from build123d import *

# Parameters (mm, degrees)
BOSS_EXTRUDE1_DEPTH      = 13.5
BOSS_EXTRUDE2_DEPTH      = 18.5
BOSS_EXTRUDE3_DEPTH      = 5
SKETCH4_W                = 45.922011884
SKETCH4_H                = 20
BOSS_EXTRUDE4_DEPTH      = 13.5
SKETCH2_R                = 4
CUT_EXTRUDE1_DEPTH       = 268.629329099
SKETCH5_R                = 8
CUT_EXTRUDE2_DEPTH       = 4
SKETCH6_R                = 9
CUT_EXTRUDE3_DEPTH       = 12
SKETCH7_R                = 12.5
CUT_EXTRUDE4_DEPTH       = 5
BOSS_EXTRUDE5_DEPTH      = 13.5
CUT_EXTRUDE5_REACH       = 210.1
CUT_EXTRUDE5_END_RADIUS  = 45
SKETCH8_R                = 9
CUT_EXTRUDE6_REACH       = 210.1
SKETCH10_R               = 4.5
SKETCH18_R               = 11
CUT_EXTRUDE9_DEPTH       = 47
CUT_EXTRUDE10_DEPTH      = 268.629329099
CUT_EXTRUDE10_DEPTH_BACK = 268.629329099
SKETCH19_W               = 45.922011884
SKETCH19_H               = 198
M6_CLEARANCE_HOLE1_D     = 6.6
SKETCH30_R               = 8.025
CUT_EXTRUDE13_DEPTH      = 4
BOSS_EXTRUDE9_DEPTH      = 16
M5_TAPPED_HOLE2_D        = 4.2
CUT_EXTRUDE16_DEPTH      = 3
M2_TAPPED_HOLE1_D        = 1.6
M2_TAPPED_HOLE1_DEPTH    = 8
M2_TAPPED_HOLE1_TIP      = 0.480688495


with BuildPart() as part:
    # Sketch1 → Boss-Extrude1 (new, symmetric)
    with BuildSketch(Plane(origin=(0, 0, 0), x_dir=(1, 0, 0), z_dir=(0, 1, 0))):
        with BuildLine():
            ThreePointArc((17.220754456, -41.574578963), (0, -45), (-17.220754456, -41.574578963))
            Line((-17.220754456, -41.574578963), (-22.961005942, -55.432771951))
            ThreePointArc((-22.961005942, -55.432771951), (0, -60), (22.961005942, -55.432771951))
            Line((22.961005942, -55.432771951), (17.220754456, -41.574578963))
        make_face()
    extrude(amount=BOSS_EXTRUDE1_DEPTH, both=True)

    # Sketch1_3 → Boss-Extrude2 (add, symmetric)
    with BuildSketch(Plane(origin=(0, 0, 0), x_dir=(1, 0, 0), z_dir=(0, 1, 0))):
        with BuildLine():
            ThreePointArc((19.134171618, -46.193976626), (0, -50), (-19.134171618, -46.193976626))
            Line((-19.134171618, -46.193976626), (-21.04758878, -50.813374288))
            ThreePointArc((-21.04758878, -50.813374288), (0, -55), (21.04758878, -50.813374288))
            Line((21.04758878, -50.813374288), (19.134171618, -46.193976626))
        make_face()
    extrude(amount=BOSS_EXTRUDE2_DEPTH, both=True)

    # Sketch3 → Boss-Extrude3 (add, symmetric)
    with BuildSketch(Plane.XZ):
        with BuildLine():
            Line((-22.961005942, 266), (-22.961005942, 55.432771951))
            ThreePointArc((-22.961005942, 55.432771951), (-20.481139434, 56.39612511), (-17.961005942, 57.248600555))
            Line((-17.961005942, 57.248600555), (-17.961005942, 246))
            Line((-17.961005942, 246), (17.961005942, 246))
            Line((17.961005942, 246), (17.961005942, 57.248600555))
            ThreePointArc((17.961005942, 57.248600555), (20.481139434, 56.39612511), (22.961005942, 55.432771951))
            Line((22.961005942, 55.432771951), (22.961005942, 266))
            Line((22.961005942, 266), (-22.961005942, 266))
        make_face()
    extrude(amount=BOSS_EXTRUDE3_DEPTH, both=True)

    # Sketch4 → Boss-Extrude4 (add, symmetric)
    with BuildSketch(Plane(origin=(0, 0, 0), x_dir=(1, 0, 0), z_dir=(0, 1, 0))):
        with Locations((0, -256)):
            Rectangle(SKETCH4_W, SKETCH4_H)
    extrude(amount=BOSS_EXTRUDE4_DEPTH, both=True)

    # Sketch2 → Cut-Extrude1 (cut, through all)
    with BuildSketch(Plane.XY):
        with Locations(Location((0, 0, 0), (0, 0, 180))):
            Circle(SKETCH2_R)
    extrude(amount=CUT_EXTRUDE1_DEPTH, mode=Mode.SUBTRACT)

    # Sketch5 → Cut-Extrude2 (cut)
    with BuildSketch(Plane(origin=(0, 0, 246), x_dir=(-1, 0, 0), z_dir=(0, 0, -1))):
        Circle(SKETCH5_R)
    extrude(amount=-CUT_EXTRUDE2_DEPTH, mode=Mode.SUBTRACT)

    # Sketch6 → Cut-Extrude3 (cut)
    with BuildSketch(Plane.XY.offset(266)):
        Circle(SKETCH6_R)
    extrude(amount=-CUT_EXTRUDE3_DEPTH, mode=Mode.SUBTRACT)

    # Sketch7 → Cut-Extrude4 (cut)
    with BuildSketch(Plane.XY.offset(266)):
        Circle(SKETCH7_R)
    extrude(amount=-CUT_EXTRUDE4_DEPTH, mode=Mode.SUBTRACT)

    # Sketch9 → Boss-Extrude5 (add, symmetric)
    with BuildSketch(Plane(origin=(0, 0, 0), x_dir=(1, 0, 0), z_dir=(0, 1, 0))):
        with BuildLine():
            Line((-22.961005942, -55.432771951), (-22.961005942, -68))
            Line((-22.961005942, -68), (22.961005942, -68))
            Line((22.961005942, -68), (22.961005942, -55.432771951))
            ThreePointArc((22.961005942, -55.432771951), (0, -60), (-22.961005942, -55.432771951))
        make_face()
    extrude(amount=BOSS_EXTRUDE5_DEPTH, both=True)

    # Cut-Extrude5: up to this cylinder (the profile starts outside it)
    cut_extrude5_end = Plane(origin=(0, 0, 0), z_dir=(0, -1, 0)) * Cylinder(CUT_EXTRUDE5_END_RADIUS, 511.2, mode=Mode.PRIVATE)
    # Sketch8 → Cut-Extrude5 (cut, up to the surface)
    with BuildSketch(Plane.XY.offset(60), mode=Mode.PRIVATE) as cut_extrude5_sk1:
        Circle(SKETCH8_R)
    cut_extrude5_tool1 = extrude(cut_extrude5_sk1.sketch, amount=-CUT_EXTRUDE5_REACH, mode=Mode.PRIVATE) - cut_extrude5_end
    add(cut_extrude5_tool1.solids().sort_by_distance((0, 0, 60))[0], mode=Mode.SUBTRACT)

    # Sketch10 → Cut-Extrude6 (cut, up to next)
    with BuildSketch(Plane.XY.offset(60), mode=Mode.PRIVATE) as cut_extrude6_sk1:
        with Locations(Location((0, 0, 0), (0, 0, 180))):
            Circle(SKETCH10_R)
    cut_extrude6_tool1 = extrude(cut_extrude6_sk1.sketch, amount=CUT_EXTRUDE6_REACH, mode=Mode.PRIVATE) & part.part
    add(cut_extrude6_tool1.solids().sort_by_distance((0, 0, 60))[0], mode=Mode.SUBTRACT)

    # Sketch18 → Cut-Extrude9 (cut)
    with BuildSketch(Plane.XY):
        with Locations(Location((0, 0, 0), (0, 0, 180))):
            Circle(SKETCH18_R)
    extrude(amount=CUT_EXTRUDE9_DEPTH, mode=Mode.SUBTRACT)

    # Sketch19 → Cut-Extrude10 (cut, two sides: drawn at the far end of the back side and taken through both)
    with BuildSketch(Plane(origin=(0, 0, 0), x_dir=(1, 0, 0), z_dir=(0, 1, 0)).offset(-CUT_EXTRUDE10_DEPTH_BACK)):
        with Locations((0, -167)):
            Rectangle(SKETCH19_W, SKETCH19_H)
    extrude(amount=CUT_EXTRUDE10_DEPTH + CUT_EXTRUDE10_DEPTH_BACK, mode=Mode.SUBTRACT)

    # Sketch23 → M5 Tapped Hole1 (revolve, cut)
    with BuildSketch(Plane(origin=(14.26606865, 8, 68), x_dir=(0, -1, 0), z_dir=(1, 0, 0))):
        Polygon((0, 0), (0, 11.3618073), (2.1, 10.1), (2.1, 0), align=None)
    m5_tapped_hole1 = revolve(axis=Axis((14.26606865, 8, 74.35), (0, 0, -1)), mode=Mode.SUBTRACT)

    # Mirror1: M5 Tapped Hole1 across plane
    add(m5_tapped_hole1.mirror(Plane(origin=(0, 0, 0), x_dir=(0, 0, 1), z_dir=(1, 0, 0))), mode=Mode.SUBTRACT)

    # M6 Clearance Hole1 (through all)
    with Locations(Plane(origin=(0, 18.5, 0), x_dir=(1, 0, 0), z_dir=(0, 1, 0))):
        with Locations((-13.587999868, -50.71110588), (13.587999868, -50.71110588)):
            Hole(M6_CLEARANCE_HOLE1_D / 2)

    # Sketch30 → Cut-Extrude13 (cut)
    with BuildSketch(Plane(origin=(0, 0, 60), x_dir=(-1, 0, 0), z_dir=(0, 0, -1))):
        Circle(SKETCH30_R)
    extrude(amount=-CUT_EXTRUDE13_DEPTH, mode=Mode.SUBTRACT)

    # Sketch37 → Boss-Extrude9 (add)
    with BuildSketch(Plane.XZ.offset(13.5)):
        with BuildLine():
            Line((-22.961005942, 68), (22.961005942, 68))
            Line((22.961005942, 68), (22.961005942, 57))
            ThreePointArc((22.961005942, 57), (0, 61.450856738), (-22.961005942, 57))
            Line((-22.961005942, 57), (-22.961005942, 68))
        make_face()
    extrude(amount=BOSS_EXTRUDE9_DEPTH)

    # M5 Tapped Hole2 (through all)
    with Locations(Plane.XY.offset(68)):
        with Locations((-14.26606865, -24), (14.26606865, -24)):
            Hole(M5_TAPPED_HOLE2_D / 2)

    # Sketch41 → Cut-Extrude16 (cut)
    with BuildSketch(Plane.XY.offset(68)):
        with BuildLine():
            Line((-7, 13.5), (-7, 8))
            ThreePointArc((-7, 8), (-6.560660172, 6.939339828), (-5.5, 6.5))
            Line((-5.5, 6.5), (5.5, 6.5))
            ThreePointArc((5.5, 6.5), (6.560660172, 6.939339828), (7, 8))
            Line((7, 8), (7, 13.5))
            Line((7, 13.5), (-7, 13.5))
        make_face()
    extrude(amount=-CUT_EXTRUDE16_DEPTH, mode=Mode.SUBTRACT)

    # M2 Tapped Hole1
    with Locations(Plane.XY.offset(65)):
        with Locations((-5, 10.5), (5, 10.5)):
            Hole(M2_TAPPED_HOLE1_D / 2, depth=M2_TAPPED_HOLE1_DEPTH)
            with Locations((0, 0, -(M2_TAPPED_HOLE1_DEPTH + M2_TAPPED_HOLE1_TIP / 2))):  # 118° drill point
                Cone(0, M2_TAPPED_HOLE1_D / 2, M2_TAPPED_HOLE1_TIP, mode=Mode.SUBTRACT)


solid = part.part
Geometry check sheet. Reference: the model listing, model coordinates, mm. A direction names the side the tool comes from. Coordinates: 2 decimals unless noted, no trailing zeros. Loops run counter-clockwise (first coordinate to the right, second up) from the corner with the lowest first, then second, coordinate; pieces in that order, holes last. Notation, with made-up numbers: (-25, 69.25) - (22, 69.25) arc R12 cw to (22, 84.25) - close; hole circle Ø1 at (73, -11.5). An arc over 180 degrees is marked (long way). Use one line per item in the form item = value. Start each with the question number.
Item 1: Section check C-C, the plane y = -6. Enter the section's corners in (x, z), and give its area (3 significant figures).
Item 2: Section check B-B, the plane y = -1. Enter the section's corners in (x, z), and give its area (3 significant figures).
Item 3: Section check D-D, the plane y = -24. Enter the section's corners in (x, z).
Item 4: Gauge pin test, flat ends, axial feed: pin 1 (10.5 mm diameter, centred on x = 0, y = 0, fed in from -Z); pin 2 (1.8 mm diameter, centred on x = -17, z = 50.5, fed in from -Y); pin 3 (4 mm diameter, centred on y = 9, z = 44.5, fed in from +X); pin 4 (5 mm diameter, centred on x = -14.27, y = -24, fed in from +Z). Record the tip position at first contact, or that the pin passes through.
Item 5: Mould release check, pull along Y, two halves, no side actions. Record for faces 1 (the face through (0, -18.5, 53)), 2 (the face through (16.364, -23.908, 63.549)), 3 (the face through (0, -16, 50)): +Y half, -Y half, draft (parallel to the pull), parting line (faces both ways), or undercut.
Item 6: Thickness scan on probe 1 along X at (y, z) = (10.5, 61); probe 2 along X at (y, z) = (-6, 48.5); probe 3 along Y at (x, z) = (5, 59.5). Record the ranges inside material, lowest first.
Item 7: Tool access check on faces 4 (the face through (6.55, 6.93, 66.52)), 5 (the face through (-2, 9, 47)), 6 (the face through (14.2, 10.1, 63)), 7 (the face through (18.687, -15.965, 51.728)). Record the directions out of +Z, -Z, +X, -X, +Y, -Y that give a thin tool (end or side, any length) a straight path to the whole face; none if there is none.
Computed:
q1.outline = (-22.96, 55.43) - (-17.22, 41.57) arc R45 cw to (-9.22, 44.05) - (-9.22, 47) - (-6.71, 47) - (-6.71, 60) - (-5.33, 60) - (-5.33, 64) - (5.33, 64) - (5.33, 60) - (6.71, 60) - (6.71, 47) - (9.22, 47) - (9.22, 44.05) arc R45 cw to (17.22, 41.57) - (22.96, 55.43) - (22.96, 68) - (-22.96, 68) - close; hole circle Ø6.6 at (-13.59, 50.71); hole circle Ø6.6 at (13.59, 50.71)
q1.area = 726 mm2
q2.outline = (-22.96, 55.43) - (-17.22, 41.57) arc R45 cw to (-10.95, 43.65) - (-10.95, 47) - (-8.94, 47) - (-8.94, 60) - (-7.96, 60) - (-7.96, 64) - (-4.39, 64) - (-4.39, 68) - (-22.96, 68) - close; (4.39, 64) - (7.96, 64) - (7.96, 60) - (8.94, 60) - (8.94, 47) - (10.95, 47) - (10.95, 43.65) arc R45 cw to (17.22, 41.57) - (22.96, 55.43) - (22.96, 68) - (4.39, 68) - close; hole circle Ø6.6 at (-13.59, 50.71); hole circle Ø6.6 at (13.59, 50.71)
q2.area = 601 mm2
q3.outline = (-22.96, 57) arc R61.45 cw to (-16.37, 59.23) - (-16.37, 68) - (-22.96, 68) - close; (-12.17, 60.23) arc R61.45 cw to (12.17, 60.23) - (12.17, 68) - (-12.17, 68) - close; (16.37, 59.23) arc R61.45 cw to (22.96, 57) - (22.96, 68) - (16.37, 68) - close
q4.pin_1 = 64
q4.pin_2 = -18.5
q4.pin_3 = 19.26
q4.pin_4 = 68
q5.face_1 = -Y half
q5.face_2 = undercut
q5.face_3 = draft
q6.probe_1 = -22.96 to -5.8, -4.2 to 4.2, 5.8 to 22.96
q6.probe_2 = -20.09 to -16.04, -11.14 to -6.71, 6.71 to 11.14, 16.04 to 20.09
q6.probe_3 = -13.5 to -7.48, 7.48 to 9.7, 11.3 to 13.5
q7.face_4 = +Z, +Y
q7.face_5 = -Z
q7.face_6 = +Z
q7.face_7 = +X, -Y
